```python
from build123d import *

# Parameters (mm, degrees)
SZKIC1_W                   = 3
SZKIC1_H                   = 19.815
SZKIC2_R                   = 3.2
WYTNIJ_WYCI_GNI_CIE1_DEPTH = 47.999650126


with BuildPart() as part:
    # Szkic1 → Obrót2 (revolve)
    with BuildSketch(Plane.XY, mode=Mode.PRIVATE) as obr_t2_sk:
        with Locations((-30.002520162, 23.2585)):
            Rectangle(SZKIC1_W, SZKIC1_H)
    revolve(obr_t2_sk.sketch.rotate(Axis((0, 0, 0), (-1, 0, 0)), 90), axis=Axis((0, 0, 0), (-1, 0, 0)))

    # Szkic2 → Wytnij-wyciągnięcie1 (cut, through all)
    with BuildSketch(Plane(origin=(-28.502520162, 0, 0), x_dir=(0, 0, -1), z_dir=(1, 0, 0))):
        with Locations((0, 27.5)):
            Circle(SZKIC2_R)
        with Locations((23.815698604, -13.75)):
            Circle(SZKIC2_R)
        with Locations((-23.815698604, -13.75)):
            Circle(SZKIC2_R)
    extrude(amount=-WYTNIJ_WYCI_GNI_CIE1_DEPTH, mode=Mode.SUBTRACT)


solid = part.part
```
Geometry: final body of the model. Coordinates: model frame, mm. Round coordinates to 2 decimals unless told otherwise and drop trailing zeros. Order: outer loops, then holes, each group sorted by start corner. A loop starts at its lowest first (then second) coordinate and runs counter-clockwise, first axis right, second up. Notation, with made-up numbers: (14, 81) -> (22, 81) arc R14 cw to (22, 89) -> close; hole circle Ø1 at (49, 61.25). An arc over 180 degrees is marked (long way). Use one line per item in the form item = value. Start each with the question number.
1. Line query: probe 1 along Y at (x, z) = (-29.5, 0); probe 2 along Y at (x, z) = (-29.3, 2.5); probe 3 along Y at (x, z) = (-30.85, -8.5). Output: solid intervals per line, ascending.
2. Cut plane C-C (z = -12.5). Return the cut outline in (x, y), then the cut area to 3 significant figures.
3. Pin query (flat end, axial travel): pin 1 Ø4 at (y, z) = (27.5, 0) entering from +X. Return the tip coordinate at first contact, or that it passes through.
4. Cut plane A-A (z = 0). Return the cut outline in (x, y).
5. Cut plane D-D (x = -30.3). Return the cut outline in (y, z), then the cut area to 3 significant figures.
6. Cut plane B-B (y = 10.5). Return the cut outline in (x, z), then the cut area to 3 significant figures.
7. Draft query along Y for faces 1 (the face through (-31.503, 0, 14)), 2 (the face through (-29.98, -22.42, 24.44)), 3 (the face through (-29.98, -16.59, 22.34)). Return one class per face: pulls with the +Y half, pulls with the -Y half, needs draft (parallel to the pull), parting line crosses it, or undercut.
Solution:
q1.probe_1 = -33.17 to -13.35, 13.35 to 24.3, 30.7 to 33.17
q1.probe_2 = -33.07 to -13.11, 13.11 to 25.5, 29.5 to 33.07
q1.probe_3 = -32.06 to -10.3, 10.3 to 32.06
q2.outline = (-31.5, -30.72) -> (-28.5, -30.72) -> (-28.5, -4.69) -> (-31.5, -4.69) -> close; (-31.5, 4.69) -> (-28.5, 4.69) -> (-28.5, 30.72) -> (-31.5, 30.72) -> close
q2.area = 156 mm^2
q3.pin_1 = through
q4.outline = (-31.5, -33.17) -> (-28.5, -33.17) -> (-28.5, -13.35) -> (-31.5, -13.35) -> close; (-31.5, 13.35) -> (-28.5, 13.35) -> (-28.5, 24.3) -> (-31.5, 24.3) -> close; (-31.5, 30.7) -> (-28.5, 30.7) -> (-28.5, 33.17) -> (-31.5, 33.17) -> close
q5.outline = circle Ø66.33 at (0, 0); hole circle Ø6.4 at (-13.75, -23.82); hole circle Ø6.4 at (-13.75, 23.82); hole circle Ø26.7 at (0, 0); hole circle Ø6.4 at (27.5, 0)
q5.area = 2,800 mm^2
q6.outline = (-31.5, -31.46) -> (-28.5, -31.46) -> (-28.5, -8.25) -> (-31.5, -8.25) -> close; (-31.5, 8.25) -> (-28.5, 8.25) -> (-28.5, 31.46) -> (-31.5, 31.46) -> close
q6.area = 139 mm^2
q7.face_1 = needs draft
q7.face_2 = parting line crosses it
q7.face_3 = undercut
